Build history of the part. All positions in model axes, mm. Round coordinates to 2 decimals unless told otherwise and drop trailing zeros. Loops run counter-clockwise (first coordinate to the right, second up) from the corner with the lowest first, then second, coordinate; pieces in that order, holes last. Notation, with made-up numbers: (26.5, 30.25) - (61.5, 30.25) arc R19 cw to (61.5, 56.25) - close; hole circle Ø2 at (63, 60). An arc over 180 degrees is marked (long way). Use one line per item in the form item = value. Start each with the question number.
Q1. Saw through at C-C (y = 13). Give the cut face in (x, z), then the cut area to 4 significant figures.
Q2. Saw through at B-B (y = -60). Give the cut face in (x, z), then the cut area to 4 significant figures.
Q3. Pin check, flat tips, straight feed: pin 1 (13 mm diameter, centred on x = 33.5, z = 411, fed in from -Y); pin 2 (12 mm diameter, centred on y = 20, z = 480.5, fed in from +X); pin 3 (6 mm diameter, centred on x = 21, z = 346.5, fed in from -Y). Stop position of each tip, or through.
Q4. Drill centre lines: line 1 (X direction, y = -4, z = 581.5); line 2 (X direction, y = -51, z = 611); line 3 (Y direction, x = 41, z = 282). Where is each one in solid material? Low to high.
Q5. Saw through at A-A (z = 589.5). Give the cut face in (x, y), then the cut area to 3 significant figures.
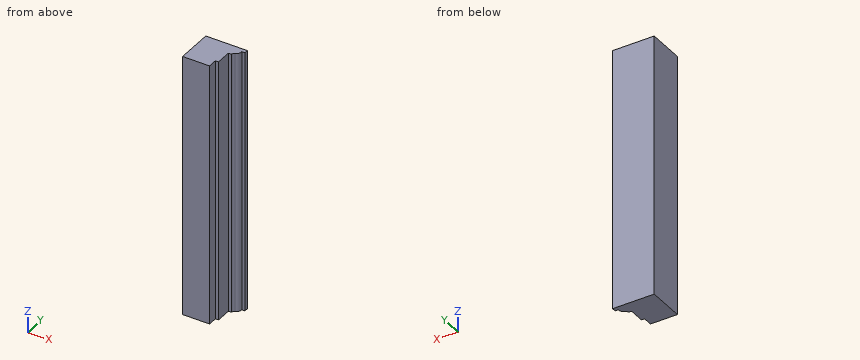
```python
from build123d import *

# Parameters (mm, degrees)
F1_DEPTH = 1000


with BuildPart() as f1:
    # F0 (on Top) → F1 (new body)
    with BuildSketch(Plane.XY):
        with BuildLine():
            Line((70.681115, 69.605961), (-87.818885, 69.605961))
            Line((-87.818885, 69.605961), (-87.818885, -70.394039))
            Line((-87.818885, -70.394039), (14.681115, -70.394039))
            Line((14.681115, -70.394039), (14.681115, -35.394039))
            Line((14.681115, -35.394039), (26.681115, -35.394039))
            Line((26.681115, -35.394039), (26.681115, 24.605961))
            Line((26.681115, 24.605961), (38.681115, 24.605961))
            ThreePointArc((38.681115, 24.605961), (40.523457, 30.389785), (45.37164, 34.042453))
            ThreePointArc((45.37164, 34.042453), (55.542724, 42.048295), (58.681115, 54.605961))
            Line((58.681115, 54.605961), (70.681115, 54.605961))
            Line((70.681115, 54.605961), (70.681115, 69.605961))
        make_face()
    extrude(amount=F1_DEPTH)


solid = f1.part
```
Report:
q1.outline = (-87.82, 0) - (26.68, 0) - (26.68, 1000) - (-87.82, 1000) - close
q1.area = 114,500 mm²
q2.outline = (-87.82, 0) - (14.68, 0) - (14.68, 1000) - (-87.82, 1000) - close
q2.area = 102,500 mm²
q3.pin_1 = 24.61
q3.pin_2 = 38.78
q3.pin_3 = -35.39
q4.line_1 = -87.82 to 26.68
q4.line_2 = -87.82 to 14.68
q4.line_3 = 31.01 to 69.61
q5.outline = (-87.82, -70.39) - (14.68, -70.39) - (14.68, -35.39) - (26.68, -35.39) - (26.68, 24.61) - (38.68, 24.61) arc R10 cw to (45.37, 34.04) arc R20 ccw to (58.68, 54.61) - (70.68, 54.61) - (70.68, 69.61) - (-87.82, 69.61) - close
q5.area = 17,000 mm²
